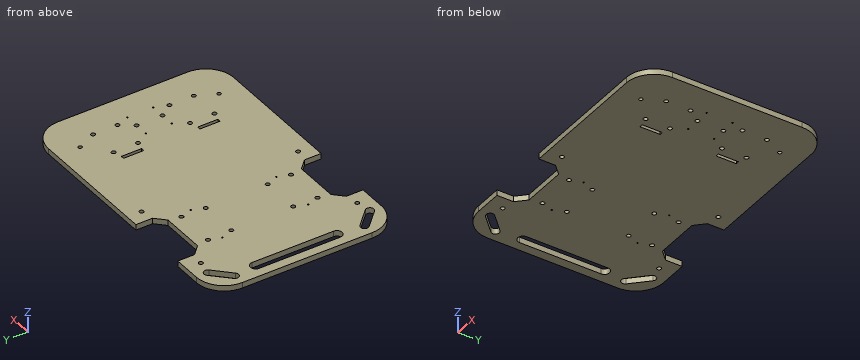
```python
from build123d import *

# Parameters (mm, degrees)
SKETCH2_R           = 2.25
SKETCH2_R_2         = 2
BOSS_EXTRUDE2_DEPTH = 6
SKETCH5_R           = 2.25
CUT_EXTRUDE2_DEPTH  = 7
SKETCH6_R           = 0.75
SKETCH6_W           = 3.570647065
SKETCH6_H           = 21.947745834
CUT_EXTRUDE3_DEPTH  = 7
SKETCH7_R           = 0.75
CUT_EXTRUDE4_DEPTH  = 7


with BuildPart() as part:
    # Sketch2 → Boss-Extrude2 (new body)
    with BuildSketch(Plane.XY):
        with BuildLine():
            ThreePointArc((0, 30), (8.786796564, 8.786796564), (30, 0))
            Line((30, 0), (60, 0))
            Line((60, 0), (60, 18))
            Line((60, 18), (70, 28))
            Line((70, 28), (118, 28))
            Line((118, 28), (128, 18))
            Line((128, 18), (128, 0))
            Line((128, 0), (270, 0))
            ThreePointArc((270, 0), (291.213203436, 8.786796564), (300, 30))
            Line((300, 30), (300, 170))
            ThreePointArc((300, 170), (291.213203436, 191.213203436), (270, 200))
            Line((270, 200), (128, 200))
            Line((128, 200), (128, 182))
            Line((128, 182), (118, 172))
            Line((118, 172), (70, 172))
            Line((70, 172), (60, 182))
            Line((60, 182), (60, 200))
            Line((60, 200), (30, 200))
            ThreePointArc((30, 200), (8.786796564, 191.213203436), (0, 170))
            Line((0, 170), (0, 30))
        make_face()
        with BuildLine():
            Line((26.918743033, 9.536510288), (9.536510288, 26.918743033))
            ThreePointArc((9.536510288, 26.918743033), (9.536510288, 32.929150673), (15.546917928, 32.929150673))
            Line((15.546917928, 32.929150673), (32.929150673, 15.546917928))
            ThreePointArc((32.929150673, 15.546917928), (32.929150673, 9.536510288), (26.918743033, 9.536510288))
        make_face(mode=Mode.SUBTRACT)
        with Locations((45.951664231, 15.546917928)):
            Circle(SKETCH2_R, mode=Mode.SUBTRACT)
        with Locations((142.048335769, 15.546917928)):
            Circle(SKETCH2_R, mode=Mode.SUBTRACT)
        with Locations((256.262155689, 25)):
            Circle(SKETCH2_R_2, mode=Mode.SUBTRACT)
        with Locations((232.877141624, 45.572368642)):
            Circle(SKETCH2_R, mode=Mode.SUBTRACT)
        with Locations((266.174553403, 45.645)):
            Circle(SKETCH2_R, mode=Mode.SUBTRACT)
        with Locations((232.771355194, 71.922156293)):
            Circle(SKETCH2_R, mode=Mode.SUBTRACT)
        with Locations((266.174553403, 71.995)):
            Circle(SKETCH2_R, mode=Mode.SUBTRACT)
        with Locations((256.262155689, 86.035)):
            Circle(SKETCH2_R, mode=Mode.SUBTRACT)
        with BuildLine():
            ThreePointArc((9.996523571, 145.539520474), (15.546917928, 151.089914831), (21.097312286, 145.539520474))
            Line((21.097312286, 145.539520474), (21.097312286, 57.620027261))
            ThreePointArc((21.097312286, 57.620027261), (15.546917928, 52.069632903), (9.996523571, 57.620027261))
            Line((9.996523571, 57.620027261), (9.996523571, 145.539520474))
        make_face(mode=Mode.SUBTRACT)
        with BuildLine():
            ThreePointArc((15.546917928, 167.070849327), (9.536510288, 167.070849327), (9.536510288, 173.081256967))
            Line((9.536510288, 173.081256967), (26.918743033, 190.463489712))
            ThreePointArc((26.918743033, 190.463489712), (32.929150673, 190.463489712), (32.929150673, 184.453082072))
            Line((32.929150673, 184.453082072), (15.546917928, 167.070849327))
        make_face(mode=Mode.SUBTRACT)
        with Locations((45.951664231, 184.453082072)):
            Circle(SKETCH2_R, mode=Mode.SUBTRACT)
        with Locations((142.048335769, 184.453082072)):
            Circle(SKETCH2_R, mode=Mode.SUBTRACT)
        with Locations((256.262155689, 113.965)):
            Circle(SKETCH2_R, mode=Mode.SUBTRACT)
        with Locations((232.771355194, 128.077843707)):
            Circle(SKETCH2_R, mode=Mode.SUBTRACT)
        with Locations((266.174553403, 128.005)):
            Circle(SKETCH2_R, mode=Mode.SUBTRACT)
        with Locations((232.877141624, 154.427631358)):
            Circle(SKETCH2_R, mode=Mode.SUBTRACT)
        with Locations((266.174553403, 154.355)):
            Circle(SKETCH2_R, mode=Mode.SUBTRACT)
        with Locations((256.262155689, 175)):
            Circle(SKETCH2_R_2, mode=Mode.SUBTRACT)
    extrude(amount=BOSS_EXTRUDE2_DEPTH)

    # Sketch5 → Cut-Extrude2 (cut, through all)
    with BuildSketch(Plane.XY.offset(6)):
        with Locations((73.27, 66.55)):
            Circle(SKETCH5_R)
        with Locations((72.45, 40.85)):
            Circle(SKETCH5_R)
        with Locations((115.55, 40.85)):
            Circle(SKETCH5_R)
        with Locations((114.73, 66.55)):
            Circle(SKETCH5_R)
        with Locations((115.55, 159.15)):
            Circle(SKETCH5_R)
        with Locations((72.45, 159.15)):
            Circle(SKETCH5_R)
        with Locations((73.27, 133.45)):
            Circle(SKETCH5_R)
        with Locations((114.73, 133.45)):
            Circle(SKETCH5_R)
    extrude(amount=-CUT_EXTRUDE2_DEPTH, mode=Mode.SUBTRACT)

    # Sketch6 → Cut-Extrude3 (cut, through all)
    with BuildSketch(Plane.XY.offset(6)):
        with Locations((68.18, 146.3)):
            Circle(SKETCH6_R)
        with Locations((119.82, 146.3)):
            Circle(SKETCH6_R)
        with Locations((119.82, 53.7)):
            Circle(SKETCH6_R)
        with Locations((68.18, 53.7)):
            Circle(SKETCH6_R)
        with Locations((221.907735921, 58.796241559)):
            Rectangle(SKETCH6_W, SKETCH6_H)
        with Locations((221.907735921, 141.203758441)):
            Rectangle(SKETCH6_W, SKETCH6_H)
    extrude(amount=-CUT_EXTRUDE3_DEPTH, mode=Mode.SUBTRACT)

    # Sketch7 → Cut-Extrude4 (cut, through all)
    with BuildSketch(Plane.XY.offset(6)):
        with Locations((241.292155689, 113.965)):
            Circle(SKETCH7_R)
        with Locations((241.292155689, 86.035)):
            Circle(SKETCH7_R)
        with Locations((271.232155689, 86.035)):
            Circle(SKETCH7_R)
        with Locations((271.232155689, 113.965)):
            Circle(SKETCH7_R)
    extrude(amount=-CUT_EXTRUDE4_DEPTH, mode=Mode.SUBTRACT)


solid = part.part
```
Here's how the part is built. I have some questions about the finished solid (model axes, mm). Round coordinates to 2 decimals unless told otherwise and drop trailing zeros. Use a Markdown table: item, result. Add a question column.
(1) Suppose I cut it at A-A, the plane z = 4.3. Count the separate pieces of the cut face and the enclosed holes in it, and give its area (3 significant figures).
(2) For pin 1 Ø1.7 at (x, y) = (241.29, 86.04) entering from +Z; pin 2 Ø1.8 at (y, z) = (10, 4) entering from -X; pin 3 Ø3 at (y, z) = (194.5, 2) entering from -X, each with a flat end and sliding along its axis, tell me the tip position at first contact or that it passes through.
(3) I need wall thicknesses on line 1 along X through (y, z) = (113, 2.85); line 2 along Y through (x, z) = (265, 2.1); line 3 along X through (y, z) = (158.5, 5.75). Which ranges of each line are inside material? Lowest first, please.
Verdict:
| question | item | result |
|---|---|---|
| 1 | separate pieces | 1 |
| 1 | enclosed holes | 37 |
| 1 | area | 53,500 mm2 |
| 2 | pin 1 | z = 6 |
| 2 | pin 2 | x = 6.87 |
| 2 | pin 3 | x = 10.74 |
| 3 | line 1 | 0 to 10, 21.1 to 254.23, 258.29 to 300 |
| 3 | line 2 | 0 to 43.73, 47.56 to 70.08, 73.91 to 126.09, 129.92 to 152.44, 156.27 to 200 |
| 3 | line 3 | 0 to 70.3, 74.6 to 113.4, 117.7 to 300 |
